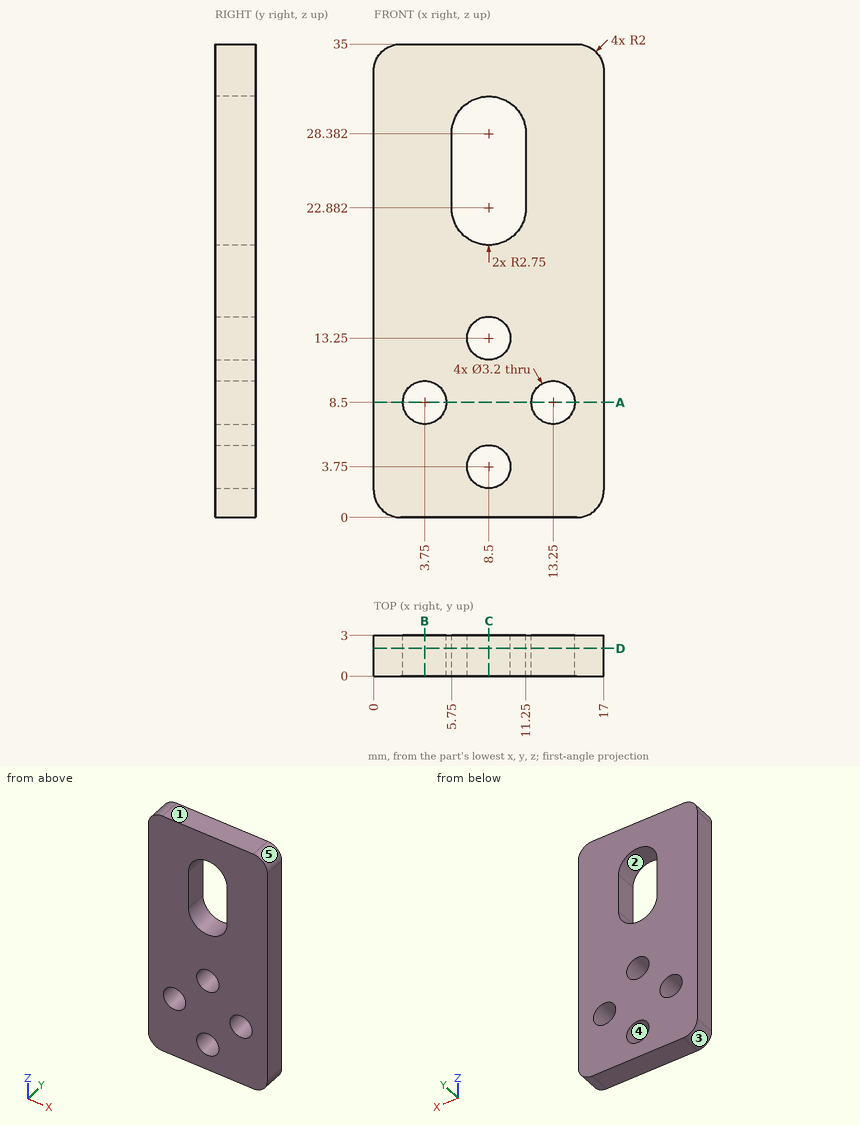
Verification items for this drawing (mm, ordinates from the low corner). A direction names the side the tool comes from. Coordinates: 2 decimals unless noted, no trailing zeros. Write each loop counter-clockwise with the first axis right and the second up, starting at its lowest first coordinate (ties: lowest second). Pieces come first, ordered by that corner, then holes. Notation, with made-up numbers: M 45,11.5 L 50,11.5 A20 cw 50,24.5 Z; hole C 33,-23.75 d9. An arc over 180 degrees is marked long. Answer as a JSON object with one key per item and string values.
1. Draft check along Z on the marked faces 3, 4 and 5. Enter one of: released by +Z, released by -Z, zero draft, split by the parting line, or undercut.
Answers below:
{"face 3": "released by -Z", "face 4": "undercut", "face 5": "released by +Z"}
2. Tool access check on the marked faces 1 and 2. Record the directions out of +Z, -Z, +X, -X, +Y, -Y that give a thin tool (end or side, any length) a straight path to the whole face; none if there is none.
Answers below:
{"face 1": "+Z, +X, -X, +Y, -Y", "face 2": "+Y, -Y"}
3. Section check D-D, the plane y = 2.05. Enter the section's corners in (x, z).
Answers below:
{"outline": "M 0,2 A2 ccw 2,0 L 15,0 A2 ccw 17,2 L 17,33 A2 ccw 15,35 L 2,35 A2 ccw 0,33 Z; hole C 3.75,8.5 d3.2; hole M 5.75,22.88 A2.75 ccw 11.25,22.88 L 11.25,28.38 A2.75 ccw 5.75,28.38 Z; hole C 8.5,3.75 d3.2; hole C 8.5,13.25 d3.2; hole C 13.25,8.5 d3.2"}
4. Section check A-A, the plane z = 8.5. Enter the section's corners in (x, y).
Answers below:
{"outline": "M 0,0 L 2.15,0 L 2.15,3 L 0,3 Z; M 5.35,0 L 11.65,0 L 11.65,3 L 5.35,3 Z; M 14.85,0 L 17,0 L 17,3 L 14.85,3 Z"}
5. Section check C-C, the plane x = 8.5. Enter the section's corners in (y, z).
Answers below:
{"outline": "M 0,0 L 3,0 L 3,2.15 L 0,2.15 Z; M 0,5.35 L 3,5.35 L 3,11.65 L 0,11.65 Z; M 0,14.85 L 3,14.85 L 3,20.13 L 0,20.13 Z; M 0,31.13 L 3,31.13 L 3,35 L 0,35 Z"}
6. Section check B-B, the plane x = 3.75. Enter the section's corners in (y, z), plus the area to 3 significant figures.
Answers below:
{"outline": "M 0,0 L 3,0 L 3,6.9 L 0,6.9 Z; M 0,10.1 L 3,10.1 L 3,35 L 0,35 Z", "area": "95.4 mm²"}
7. Scan lines: L1, parallel to X at y = 1.85, z = 8.5; L2, parallel to Z at x = 8.5, y = 1.05; L3, parallel to X at y = 1.8, z = 3.75. Record each from-to range of solid material in increasing order.
Answers below:
{"L1": "x = 0 to 2.15, 5.35 to 11.65, 14.85 to 17", "L2": "z = 0 to 2.15, 5.35 to 11.65, 14.85 to 20.13, 31.13 to 35", "L3": "x = 0 to 6.9, 10.1 to 17"}
8. Go/stop test with a flat-tipped pin: pin 1 Ø3 at (x, z) = (8.5, 13.25) entering from +Y. Record where the tip stops, or that it passes through.
Answers below:
{"pin 1": "passes through"}
